from build123d import *

# Parameters (mm, degrees)
F0_R        = 40
F1_DEPTH    = 3
F2_R        = 28
F3_DEPTH    = 16
F4_R        = 25
F5_DEPTH    = 16
F6_R        = 28
F6_R_2      = 1.75
F7_DEPTH    = 4
F8_T1_DEPTH = 4
F8_T3_DEPTH = 19
F9_R        = 4
F10_DEPTH   = 19
F13_W       = 24
F13_H       = 16
F14_DEPTH   = 84.5695424949
F16_W       = 24
F16_H       = 16
F17_DEPTH   = 84.5695424949
F18_R       = 1.3
F19_DEPTH   = 3.001
F20_R       = 2.5
F20_R_2     = 1.3088878735
F21_DEPTH   = 3
F23_DEPTH   = 3
F24_R       = 5


# Not quite as in the source:
# - a fillet or chamfer that OpenCascade refuses, or shapes differently, is made with other operations: its cross-section is extruded or revolved along the edge and cut away or added
# - an extrude ends at something that could not be found from the text; its depth is read off the source's solid


with BuildPart() as f1:
    # F0 (on Top) → F1 (new body)
    with BuildSketch(Plane.XY):
        Circle(F0_R)
    extrude(amount=F1_DEPTH)

    # F2 (on face) → F3 (join)
    with BuildSketch(Plane.XY.offset(3)):
        Circle(F2_R)
    extrude(amount=F3_DEPTH)

    # F4 (on face) → F5 (cut)
    with BuildSketch(Plane.XY.offset(19)):
        Circle(F4_R)
    extrude(amount=-F5_DEPTH, mode=Mode.SUBTRACT)

    # F6 (on face) → F7 (join)
    with BuildSketch(Plane.XY.offset(19)):
        Circle(F6_R)
        with BuildLine():
            ThreePointArc((-5, 24.4948974278), (0, 25), (5, 24.4948974278))
            ThreePointArc((5, 24.4948974278), (17.6776695297, 17.6776695297), (24.4948974278, 5))
            ThreePointArc((24.4948974278, 5), (24.8734038251, 2.5127240501), (25, 0))
            ThreePointArc((25, 0), (24.8734038251, -2.5127240501), (24.4948974278, -5))
            ThreePointArc((24.4948974278, -5), (17.6776695297, -17.6776695297), (5, -24.4948974278))
            ThreePointArc((5, -24.4948974278), (0, -25), (-5, -24.4948974278))
            ThreePointArc((-5, -24.4948974278), (-17.6776695297, -17.6776695297), (-24.4948974278, -5))
            ThreePointArc((-24.4948974278, -5), (-25, 0), (-24.4948974278, 5))
            ThreePointArc((-24.4948974278, 5), (-17.6776695297, 17.6776695297), (-5, 24.4948974278))
        make_face(mode=Mode.SUBTRACT)
        with BuildLine():
            Line((-17, 5), (-24.4948974278, 5))
            ThreePointArc((-24.4948974278, 5), (-25, 0), (-24.4948974278, -5))
            Line((-24.4948974278, -5), (-17, -5))
            Line((-17, -5), (-17, 5))
        make_face()
        with Locations((-22, 0)):
            Circle(F6_R_2, mode=Mode.SUBTRACT)
        with BuildLine():
            Line((-5, 17), (5, 17))
            Line((5, 17), (5, 24.4948974278))
            ThreePointArc((5, 24.4948974278), (0, 25), (-5, 24.4948974278))
            Line((-5, 24.4948974278), (-5, 17))
        make_face()
        with Locations((0, 22)):
            Circle(F6_R_2, mode=Mode.SUBTRACT)
        with BuildLine():
            ThreePointArc((25, 0), (24.8734038251, 2.5127240501), (24.4948974278, 5))
            Line((24.4948974278, 5), (17, 5))
            Line((17, 5), (17, -5))
            Line((17, -5), (24.4948974278, -5))
            ThreePointArc((24.4948974278, -5), (24.8734038251, -2.5127240501), (25, 0))
        make_face()
        with Locations((22, 0)):
            Circle(F6_R_2, mode=Mode.SUBTRACT)
        with BuildLine():
            Line((-5, -17), (-5, -24.4948974278))
            ThreePointArc((-5, -24.4948974278), (0, -25), (5, -24.4948974278))
            Line((5, -24.4948974278), (5, -17))
            Line((5, -17), (-5, -17))
        make_face()
        with Locations((0, -22)):
            Circle(F6_R_2, mode=Mode.SUBTRACT)
    extrude(amount=F7_DEPTH)

    # F8: fillet of radius 3 on 16 edges, made by hand

    # F8_s2 → F8_t1 (join)
    with BuildSketch(Plane.XY.offset(19)):
        with BuildLine():
            ThreePointArc((9.0909090909, 23.2885244681), (6.3077717755, 22.9710700035), (5, 20.4939015319))
            Line((5, 20.4939015319), (5, 24.4948974278))
            ThreePointArc((5, 24.4948974278), (7.0712278765, 23.9791104155), (9.0909090909, 23.2885244681))
        make_face()
        with BuildLine():
            ThreePointArc((-5, 20.4939015319), (-6.3077717755, 22.9710700035), (-9.0909090909, 23.2885244681))
            ThreePointArc((-9.0909090909, 23.2885244681), (-7.0712278765, 23.9791104155), (-5, 24.4948974278))
            Line((-5, 24.4948974278), (-5, 20.4939015319))
        make_face()
        with BuildLine():
            ThreePointArc((-23.2885244681, 9.0909090909), (-22.9710700035, 6.3077717755), (-20.4939015319, 5))
            Line((-20.4939015319, 5), (-24.4948974278, 5))
            ThreePointArc((-24.4948974278, 5), (-23.9791104155, 7.0712278765), (-23.2885244681, 9.0909090909))
        make_face()
        with BuildLine():
            ThreePointArc((-23.2885244681, -9.0909090909), (-22.9710700035, -6.3077717755), (-20.4939015319, -5))
            Line((-20.4939015319, -5), (-24.4948974278, -5))
            ThreePointArc((-24.4948974278, -5), (-23.9791104155, -7.0712278765), (-23.2885244681, -9.0909090909))
        make_face()
        with BuildLine():
            ThreePointArc((20.4939015319, 5), (22.9710700035, 6.3077717755), (23.2885244681, 9.0909090909))
            ThreePointArc((23.2885244681, 9.0909090909), (23.9791104155, 7.0712278765), (24.4948974278, 5))
            Line((24.4948974278, 5), (20.4939015319, 5))
        make_face()
        with BuildLine():
            ThreePointArc((23.2885244681, -9.0909090909), (22.9710700035, -6.3077717755), (20.4939015319, -5))
            Line((20.4939015319, -5), (24.4948974278, -5))
            ThreePointArc((24.4948974278, -5), (23.9791104155, -7.0712278765), (23.2885244681, -9.0909090909))
        make_face()
        with BuildLine():
            ThreePointArc((-9.0909090909, -23.2885244681), (-6.3077717755, -22.9710700035), (-5, -20.4939015319))
            Line((-5, -20.4939015319), (-5, -24.4948974278))
            ThreePointArc((-5, -24.4948974278), (-7.0712278765, -23.9791104155), (-9.0909090909, -23.2885244681))
        make_face()
        with BuildLine():
            ThreePointArc((5, -20.4939015319), (6.3077717755, -22.9710700035), (9.0909090909, -23.2885244681))
            ThreePointArc((9.0909090909, -23.2885244681), (7.0712278765, -23.9791104155), (5, -24.4948974278))
            Line((5, -24.4948974278), (5, -20.4939015319))
        make_face()
    extrude(amount=F8_T1_DEPTH)

    # F8_s4 → F8_t3 (cut)
    with BuildSketch(Plane.XY.offset(11.5)):
        with BuildLine():
            ThreePointArc((-17, -2), (-17.8786796564, -4.1213203436), (-20, -5))
            Line((-20, -5), (-17, -5))
            Line((-17, -5), (-17, -2))
        make_face()
        with BuildLine():
            ThreePointArc((-20, 5), (-17.8786796564, 4.1213203436), (-17, 2))
            Line((-17, 2), (-17, 5))
            Line((-17, 5), (-20, 5))
        make_face()
        with BuildLine():
            ThreePointArc((-2, 17), (-4.1213203436, 17.8786796564), (-5, 20))
            Line((-5, 20), (-5, 17))
            Line((-5, 17), (-2, 17))
        make_face()
        with BuildLine():
            ThreePointArc((5, 20), (4.1213203436, 17.8786796564), (2, 17))
            Line((2, 17), (5, 17))
            Line((5, 17), (5, 20))
        make_face()
        with BuildLine():
            ThreePointArc((20, -5), (17.8786796564, -4.1213203436), (17, -2))
            Line((17, -2), (17, -5))
            Line((17, -5), (20, -5))
        make_face()
        with BuildLine():
            ThreePointArc((17, 2), (17.8786796564, 4.1213203436), (20, 5))
            Line((20, 5), (17, 5))
            Line((17, 5), (17, 2))
        make_face()
        with BuildLine():
            ThreePointArc((2, -17), (4.1213203436, -17.8786796564), (5, -20))
            Line((5, -20), (5, -17))
            Line((5, -17), (2, -17))
        make_face()
        with BuildLine():
            ThreePointArc((-5, -20), (-4.1213203436, -17.8786796564), (-2, -17))
            Line((-2, -17), (-5, -17))
            Line((-5, -17), (-5, -20))
        make_face()
    extrude(amount=F8_T3_DEPTH, mode=Mode.SUBTRACT)

    # F9 (on face) → F10 (cut, through all)
    with BuildSketch(Plane(origin=(0, 0, 0), x_dir=(1, 0, 0), z_dir=(0, 0, -1))):
        with Locations((0, 22)):
            Circle(F9_R)
        with Locations((-22, 0)):
            Circle(F9_R)
        with Locations((0, -22)):
            Circle(F9_R)
        with Locations((22, 0)):
            Circle(F9_R)
    extrude(amount=-F10_DEPTH, mode=Mode.SUBTRACT)

    # F13 (on line) → F14 (cut, through all)
    with BuildSketch(Plane(origin=(-19.7989898732, -19.7989898732, 0), x_dir=(0.7071067812, -0.7071067812, 0), z_dir=(-0.7071067812, -0.7071067812, 0))):
        with Locations((0, 11)):
            Rectangle(F13_W, F13_H)
    extrude(amount=-F14_DEPTH, mode=Mode.SUBTRACT)

    # F16 (on line) → F17 (cut, through all)
    with BuildSketch(Plane(origin=(-19.7989898732, 19.7989898732, 0), x_dir=(-0.7071067812, -0.7071067812, 0), z_dir=(-0.7071067812, 0.7071067812, 0))):
        with Locations((0, 11)):
            Rectangle(F16_W, F16_H)
    extrude(amount=-F17_DEPTH, mode=Mode.SUBTRACT)

    # F18 (on face) → F19 (cut, through all)
    with BuildSketch(Plane.XY.offset(3)):
        with Locations((-9, 5.5)):
            Circle(F18_R)
        with Locations((9, 5.5)):
            Circle(F18_R)
        with Locations((9, -5.5)):
            Circle(F18_R)
        with Locations((-9, -5.5)):
            Circle(F18_R)
    extrude(amount=-F19_DEPTH, mode=Mode.SUBTRACT)

    # F20 (on face) → F21 (join)
    with BuildSketch(Plane.XY.offset(3)):
        with Locations((-9, 5.5)):
            Circle(F20_R)
        with Locations((-9, 5.5)):
            Circle(F20_R_2, mode=Mode.SUBTRACT)
        with Locations((9, 5.5)):
            Circle(F20_R)
        with Locations((9, 5.5)):
            Circle(F20_R_2, mode=Mode.SUBTRACT)
        with Locations((-9, -5.5)):
            Circle(F20_R)
        with Locations((-9, -5.5)):
            Circle(F20_R_2, mode=Mode.SUBTRACT)
        with Locations((9, -5.5)):
            Circle(F20_R)
        with Locations((9, -5.5)):
            Circle(F20_R_2, mode=Mode.SUBTRACT)
    extrude(amount=F21_DEPTH)

    # F22 (on face) → F23 (cut, through all)
    with BuildSketch(Plane(origin=(0, 0, 0), x_dir=(1, 0, 0), z_dir=(0, 0, -1))):
        with BuildLine():
            Line((-9.9123141263, 9.9123141263), (-9.9123141263, 34.1129360408))
            ThreePointArc((-9.9123141263, 34.1129360408), (-18.0837856402, 30.5765117954), (-25.1191796906, 25.1191796906))
            Line((-25.1191796906, 25.1191796906), (-9.9123141263, 9.9123141263))
        make_face()
        with BuildLine():
            Line((-9.9123141263, 9.9123141263), (-25.1191796906, 25.1191796906))
            ThreePointArc((-25.1191796906, 25.1191796906), (-30.5765117954, 18.0837856402), (-34.1129360408, 9.9123141263))
            Line((-34.1129360408, 9.9123141263), (-9.9123141263, 9.9123141263))
        make_face()
        with BuildLine():
            Line((9.9123141263, 9.9123141263), (34.1129360408, 9.9123141263))
            ThreePointArc((34.1129360408, 9.9123141263), (25.1191796906, 25.1191796906), (9.9123141263, 34.1129360408))
            Line((9.9123141263, 34.1129360408), (9.9123141263, 9.9123141263))
        make_face()
        with BuildLine():
            ThreePointArc((9.9123141263, -34.1129360408), (25.1191796906, -25.1191796906), (34.1129360408, -9.9123141263))
            Line((34.1129360408, -9.9123141263), (9.9123141263, -9.9123141263))
            Line((9.9123141263, -9.9123141263), (9.9123141263, -34.1129360408))
        make_face()
        with BuildLine():
            ThreePointArc((-34.1129360408, -9.9123141263), (-25.1191796906, -25.1191796906), (-9.9123141263, -34.1129360408))
            Line((-9.9123141263, -34.1129360408), (-9.9123141263, -9.9123141263))
            Line((-9.9123141263, -9.9123141263), (-34.1129360408, -9.9123141263))
        make_face()
    extrude(amount=-F23_DEPTH, mode=Mode.SUBTRACT)

    # F24
    f24_edges = [f1.edges().sort_by_distance(p)[0] for p in [
        (9.912314, 9.912314, 1.5),
        (9.912314, -9.912314, 1.5),
        (-9.912314, 9.912314, 1.5),
        (-9.912314, -9.912314, 1.5),
    ]]
    fillet(f24_edges, radius=F24_R)


solid = f1.part
Read the model definition and answer for the solid it produces. Units are mm, in the model's axes. A direction names the side the tool comes from. Give positions to 0.01 mm unless a question says otherwise; leave off trailing zeros. Write each loop counter-clockwise with the first axis right and the second up, starting at its lowest first coordinate (ties: lowest second). Pieces come first, ordered by that corner, then holes. Notation, with made-up numbers: M 41.5,-7.5 L 99.5,-7.5 A25 cw 99.5,26.5 Z; hole C 54,42.5 d7. An arc over 180 degrees is marked long. One line per item, written item: value. Start each with the question number.
(1) Find the intervals of material crossed by line 1 (X direction, y = 0, z = 9.25); line 2 (X direction, y = -21.5, z = 21); line 3 (Z direction, x = -20.5, y = 33.5), in increasing order.
(2) Find section C-C (y = 11.5). Determine the outline of the cut face in (x, z), plus the area to 3 significant figures.
(3) Determine the mould class of faces 5 (the flat face through (-25.2, 8.23, 10.89)), 6 (the cylindrical face through (-26, 0, 7)), 7 (the flat face through (-25.2, -8.23, 10.89)) for opening direction Y: pulls with the +Y half, pulls with the -Y half, needs draft (parallel to the pull), parting line crosses it, or undercut.
(4) Find section A-A (z = 14). Determine the outline of the cut face in (x, y).
(5) Find section D-D (x = -22). Give the number of separate pieces and of enclosed holes in the cut face, plus the area to 3 significant figures.
(6) Flat-ended cylindrical pins translate along their axes: pin 1 Ø5 at (y, z) = (3.5, 7) entering from +X; pin 2 Ø3 at (x, y) = (-23, -0.5) entering from -Z; pin 3 Ø3.5 at (x, y) = (9, 5.5) entering from +Z; pin 4 Ø2.5 at (x, y) = (-9, 5.5) entering from +Z. Find the tip coordinate at first contact, or state that the pin passes through.
(7) Find section B-B (x = -30). Determine the outline of the cut face in (y, z), plus the area to 3 significant figures.
(8) A tool of negligible diameter and unlimited length cuts with its end or side. For faces 1 (the flat face through (-8.23, 25.2, 10.89)), 2 (the cylindrical face through (-6.274, 22.948, 20.972)), 3 (the cylindrical face through (-8.67, -39.05, 1.48)), 4 (the flat face through (18, 2, 19)), from which of +Z, -Z, +X, -X, +Y, -Y can it reach the whole face along a straight path? Write none if from no direction.
Results below:
1. line 1: x = -28 to -26, 26 to 28
1. line 2: x = -17.94 to -12.76, -5.17 to -1.68, 1.68 to 5.17, 12.76 to 17.94
1. line 3: z = 0 to 3
2. outline: M -38.31,0 L -33.61,0 L -33.61,3 L -38.31,3 Z; M -25.53,19 L -22.2,19 L -22.2,23 L -25.53,23 Z; M -11.26,0 L 11.26,0 L 11.26,3 L -11.26,3 Z; M 22.2,19 L 25.53,19 L 25.53,23 L 22.2,23 Z; M 33.61,0 L 38.31,0 L 38.31,3 L 33.61,3 Z
2. area: 122 mm^2
3. face 5: pulls with the +Y half
3. face 6: undercut
3. face 7: pulls with the -Y half
4. outline: M -26.37,-9.4 L -23.99,-7.02 A25 cw -24.84,-2.82 A4 cw -24.84,2.82 A25 cw -23.99,7.02 L -26.37,9.4 A28 ccw Z; M -9.4,-26.37 A28 ccw 9.4,-26.37 L 7.02,-23.99 A25 cw 2.82,-24.84 A4 cw -2.82,-24.84 A25 cw -7.02,-23.99 Z; M -9.4,26.37 L -7.02,23.99 A25 cw -2.82,24.84 A4 cw 2.82,24.84 A25 cw 7.02,23.99 L 9.4,26.37 A28 ccw Z; M 23.99,-7.02 L 26.37,-9.4 A28 ccw 26.37,9.4 L 23.99,7.02 A25 cw 24.84,2.82 A4 cw 24.84,-2.82 A25 cw Z
5. separate pieces: 8
5. enclosed holes: 0
5. area: 141 mm^2
6. pin 1: stops at x = 27.98
6. pin 2: stops at z = 19
6. pin 3: stops at z = 6
6. pin 4: passes through
7. outline: M -26.46,0 L -19.02,0 L -19.02,3 L -26.46,3 Z; M -9.91,0 L 9.91,0 L 9.91,3 L -9.91,3 Z; M 19.02,0 L 26.46,0 L 26.46,3 L 19.02,3 Z
7. area: 104 mm^2
8. face 1: -X
8. face 2: +Z
8. face 3: +Z, -Z
8. face 4: none
